from build123d import *

# Parameters (mm, degrees)
CORTE_EXTERIOR_R        = 3.500001168
SALIENTE_EXTRUIR1_DEPTH = 3
CORTAR_EXTRUIR1_DEPTH   = 1


with BuildPart() as part:
    # Corte exterior → Saliente-Extruir1 (new body)
    with BuildSketch(Plane.XY):
        with BuildLine():
            Line((31.389373952, 4.705371802), (72.389373952, 4.705371802))
            ThreePointArc((72.389373952, 4.705371802), (81.389373952, 13.705371802), (72.389373952, 22.705371802))
            Line((72.389373952, 22.705371802), (31.389373952, 22.705371802))
            ThreePointArc((31.389373952, 22.705371802), (22.389373952, 13.705371802), (31.389373952, 4.705371802))
        make_face()
        with Locations((72.389373952, 13.705371802)):
            Circle(CORTE_EXTERIOR_R, mode=Mode.SUBTRACT)
    extrude(amount=SALIENTE_EXTRUIR1_DEPTH)

    # Grabado Superficie → Cortar-Extruir1 (cut)
    with BuildSketch(Plane.XY):
        with BuildLine():
            Line((70.385171574, 16.57472382), (57.998553299, 15.700408028))
            ThreePointArc((57.998553299, 15.700408028), (56.139373952, 13.705371802), (57.998553299, 11.710335575))
            Line((57.998553299, 11.710335575), (70.385171574, 10.836019783))
            ThreePointArc((70.385171574, 10.836019783), (68.889372784, 13.705371802), (70.385171574, 16.57472382))
        make_face()
    extrude(amount=CORTAR_EXTRUIR1_DEPTH, mode=Mode.SUBTRACT)


solid = part.part
Source: CAD feature listing. Evaluate the final solid. Frame: model axes, mm. A direction names the side the tool comes from. Coordinates: 2 decimals unless noted, no trailing zeros. Order: outer loops, then holes, each group sorted by start corner. A loop starts at its lowest first (then second) coordinate and runs counter-clockwise, first axis right, second up. Notation, with made-up numbers: M 86.5,69.25 L 97.5,69.25 A22 ccw 97.5,104.25 Z; hole C 7.25,89.25 d7. An arc over 180 degrees is marked long. Write each question's results on one line, items separated by ' | '. Start each with the question number.
1. Pin query (flat end, axial travel): pin 1 (1 mm diameter, centred on y = 8.5, z = 2.5, fed in from +X); pin 2 (1.5 mm diameter, centred on y = 19.5, z = 1, fed in from -X). Return the tip coordinate at first contact, or that it passes through.
2. Section B-B, the plane x = 57.5. Return the cut outline in (y, z).
3. Material intervals for L1, parallel to X at y = 16.75, z = 1.35; L2, parallel to Y at x = 57.5, z = 0.5; L3, parallel to X at y = 15.5, z = 0.95, sorted ascending.
4. Draft query along X for faces 1 (the face through (56.14, 13.75, 0.49)), 2 (the face through (51, 14, 3)), 3 (the face through (81.387, 13.507, 1.479)). Return one class per face: +X half, -X half, draft (parallel to the pull), parting line (faces both ways), or undercut.
5. Reachability of faces 4 (the face through (52, 22.705, 1)), 5 (the face through (64.11, 11.28, 0.49)) from +Z, -Z, +X, -X, +Y, -Y: full face, straight path, thin tool, end or side. Return the list, or none.
6. Section C-C, the plane z = 2.25. Return the cut outline in (x, y).
7. Section D-D, the plane y = 6.5. Return the cut outline in (x, z), then the cut area to 3 significant figures.
8. Section A-A, the plane y = 12.75. Return the cut outline in (x, z).
Solution:
1) pin 1: x = 80.06 | pin 2: x = 23.94
2) outline: M 4.71,0 L 11.81,0 L 11.81,1 L 15.6,1 L 15.6,0 L 22.71,0 L 22.71,3 L 4.71,3 Z
3) L1: 22.92 to 70.66, 74.12 to 80.86 | L2: 4.71 to 11.81, 15.6 to 22.71 | L3: 22.57 to 57.26, 75.39 to 81.21
4) face 1: undercut | face 2: draft | face 3: +X half
5) face 4: +Z, -Z, +X, -X, +Y | face 5: -Z
6) outline: M 31.39,4.71 L 72.39,4.71 A9 ccw 72.39,22.71 L 31.39,22.71 A9 ccw Z; hole C 72.39,13.71 d7
7) outline: M 26,0 L 77.78,0 L 77.78,3 L 26,3 Z | area: 155 mm²
8) outline: M 22.44,0 L 56.38,0 L 56.38,1 L 69.02,1 L 69.02,3 L 22.44,3 Z; M 75.76,0 L 81.34,0 L 81.34,3 L 75.76,3 Z
